Verification items for the finished model (mm, model axes). Round coordinates to 2 decimals unless told otherwise and drop trailing zeros. Loops run counter-clockwise (first coordinate to the right, second up) from the corner with the lowest first, then second, coordinate; pieces in that order, holes last. Notation, with made-up numbers: (81, 30.25) -> (87, 30.25) arc R13 ccw to (87, 53.25) -> close; hole circle Ø10 at (3, 42.25). An arc over 180 degrees is marked (long way). Write item = value, one per line.
Autodesk Inventor part; units mm, degrees
ref_plane "YZ Plane" through (0, 0, 0) normal (1, 0, 0) x (0, 1, 0)
ref_plane "XZ Plane" through (0, 0, 0) normal (0, 1, 0) x (-1, 0, 0)
ref_plane "XY Plane" through (0, 0, 0) normal (0, 0, 1) x (1, 0, 0)
sketch "Sketch1" plane through (0, 0, 0) normal (0, 0, 1) x (1, 0, 0)
  line L0 (0, 0) -> (-110, 0)
  line L1 (-110, 0) -> (-110, 110)
  line L2 (-110, 110) -> (0, 110)
  line L3 (0, 110) -> (0, 0)
  dimension "pcb_size" = 110
  dimension "d1" = 110
extrude "Extrusion1" add sketch "Sketch1" along normal blind 1.6
fillet "Fillet1" radius 4 4 edges at (0, 0, 0.8) (0, 110, 0.8) (-110, 110, 0.8) (-110, 0, 0.8)
sketch "Sketch2" plane through (0, 0, 1.6) normal (0, 0, 1) x (1, 0, 0)
  line L0 (0, 4) -> (0, 106)
  line L1 (-4, 110) -> (-106, 110)
  line L2 (-55, 110) -> (-55, 0) construction
  line L3 (-106, 0) -> (-4, 0) construction
  line L4 (0, 55) -> (-110, 55) construction
  line L5 (-110, 106) -> (-110, 4) construction
  point P0 (0, 0)
  point P1 (-6, 104)
  point P2 (-104, 104)
  point P3 (-6, 6)
  point P4 (-104, 6)
  dimension "d12" = 6
  dimension "d13" = 6
  dimension "pcb_fixation_ecart" = 98
  dimension "d28" = 98
hole "Hole1" at (-6, 104, 1.6) at (-6, 6, 1.6) at (-104, 6, 1.6) at (-104, 104, 1.6) direction (0, 0, -1) diameter 4.5 end through all
sketch "Sketch3" plane through (-55, 69.5861, 1.6) normal (0, 0, 1) x (1, 0, 0)
  line L0 (-24.5, -47.5861) -> (24.5, -47.5861) construction
  line L1 (-24.5, -47.5861) -> (-24.5, 10.4139) construction
  line L2 (0, -47.5861) -> (0, 10.4139) construction
  line L3 (-24.5, 10.4139) -> (24.5, 10.4139) construction
  line L4 (24.5, 10.4139) -> (24.5, -47.5861) construction
  line L5 (0, -4) -> (-24.5, -47.5861) construction
  line L6 (55, -65.5861) -> (55, 36.4139)
  line L7 (-55, 36.4139) -> (-55, -65.5861)
  line L8 (51, 40.4139) -> (-51, 40.4139)
  dimension "d16" = 58
  dimension "d15" = 49
  dimension "d17" = 50
  dimension "d24" = 110
  dimension "d25" = 55
  dimension "d26" = 30
hole "Hole2" at (-79.5, 22, 1.6) at (-79.5, 80, 1.6) at (-30.5, 22, 1.6) at (-30.5, 80, 1.6) direction (0, 0, -1) diameter 2.9 end through all
equation "\"d25\" = 0.5 * d24"
properties part number "pcb"
(1) Draft check along X on faces 1 (the face through (-1.141, 108.797, 0.811)), 2 (the face through (-101.804, 6.488, 0.789)), 3 (the face through (-108.797, 108.859, 0.811)), 4 (the face through (-6.676, 3.854, 0.789)). Enter one of: released by +X, released by -X, zero draft, split by the parting line, or undercut.
Filled sheet:
face_1 = released by +X
face_2 = undercut
face_3 = released by -X
face_4 = undercut
(2) Go/stop test with flat-tipped pins: pin 1 Ø4 at (x, y) = (-104, 104) entering from -Z; pin 2 Ø3.5 at (x, y) = (-30.5, 80) entering from -Z. Record where each tip stops, or that it passes through.
Filled sheet:
pin_1 = through
pin_2 = 0
(3) Material ranges on probe 1 along Y at (x, z) = (-6, 1.15); probe 2 along X at (y, z) = (80, 0.55); probe 3 along X at (y, z) = (6, 0.6), recorded low to high. Write a range as from..to.
Filled sheet:
probe_1 = 0..3.75, 8.25..101.75, 106.25..110
probe_2 = -110..-80.95, -78.05..-31.95, -29.05..0
probe_3 = -110..-106.25, -101.75..-8.25, -3.75..0
(4) Sectioned sample at B-B, the plane x = -6. Record the cut outline in (y, z).
Filled sheet:
outline = (0, 0) -> (3.75, 0) -> (3.75, 1.6) -> (0, 1.6) -> close; (8.25, 0) -> (101.75, 0) -> (101.75, 1.6) -> (8.25, 1.6) -> close; (106.25, 0) -> (110, 0) -> (110, 1.6) -> (106.25, 1.6) -> close
(5) Sectioned sample at A-A, the plane y = 104. Record the cut outline in (x, z), and give its area (3 significant figures).
Filled sheet:
outline = (-110, 0) -> (-106.25, 0) -> (-106.25, 1.6) -> (-110, 1.6) -> close; (-101.75, 0) -> (-8.25, 0) -> (-8.25, 1.6) -> (-101.75, 1.6) -> close; (-3.75, 0) -> (0, 0) -> (0, 1.6) -> (-3.75, 1.6) -> close
area = 162 mm2
